Source: CAD feature listing. Evaluate the final solid. Frame: model axes, mm. Face numbers are marked on the shaded views. A direction names the side the tool comes from. Give positions to 0.01 mm unless a question says otherwise; leave off trailing zeros. Order: outer loops, then holes, each group sorted by start corner. A loop starts at its lowest first (then second) coordinate and runs counter-clockwise, first axis right, second up.
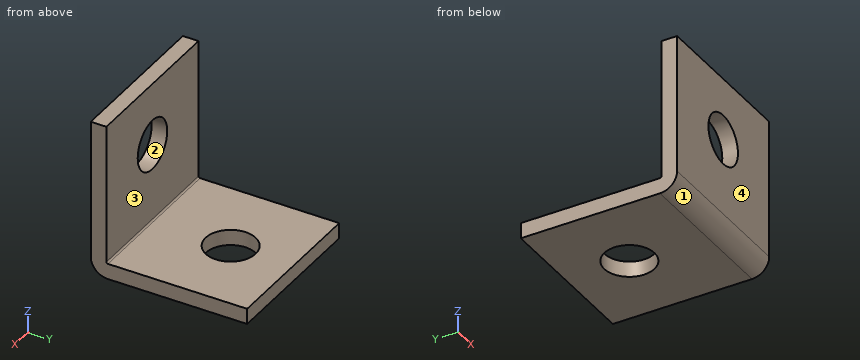
Autodesk Inventor part; units mm, degrees
ref_plane "YZ Plane" through (0, 0, 0) normal (1, 0, 0) x (0, 1, 0)
ref_plane "XZ Plane" through (0, 0, 0) normal (0, 1, 0) x (-1, 0, 0)
ref_plane "XY Plane" through (0, 0, 0) normal (0, 0, 1) x (1, 0, 0)
sketch "Sketch1" plane through (0, 0, 0) normal (0, 0, 1) x (1, 0, 0)
  line L0 (-5, 5) -> (5, 5)
  line L1 (5, 5) -> (5, -5)
  line L2 (5, -5) -> (-5, -5)
  line L3 (-5, -5) -> (-5, 5)
  line L4 (-5, 5) -> (5, -5) construction
  line L5 (5, 5) -> (-5, -5) construction
  circle A0 centre (0, 1) radius 1.6
  point P0 (0, 0)
  dimension "d0" = 10
  dimension "d1" = 10
  dimension "d3" = 3.2
  dimension "d21" = 4
extrude "Plate1" add sketch "Sketch1" along normal blind 1
sketch "Sketch2" plane through (5, -4, 0) normal (0, -1, 0) x (1, 0, 0)
  line L0 (-10, 0) -> (0, 0)
  line L1 (0, 0) -> (0, 10)
  line L2 (0, 10) -> (-10, 10)
  line L3 (-10, 10) -> (-10, 0)
edge flange "Flange1" height 10 angle 90 thickness 1 bend radius 0.1 thickness toward (0, -1, 0) relief tear relief width 1 relief depth 0.5 edges at (0, -5, 1) wall of the first edge with corners at (-5, -4, 0) (5, -4, 0) (5, -4, 10) (-5, -4, 10)
bend "Bend1"
corner "Corner1"
sketch "Sketch3" plane through (-5, -4, 10) normal (0, 1, 0) x (1, 0, 0)
  circle A0 centre (5, 4) radius 1.6
  line L0 (0, 9) -> (10, 9)
  line L1 (0, 0) -> (10, 0)
  point P0 (5, 10)
  point P1 (5, 0)
  dimension "d17" = 3.2
  dimension "d22" = 4
extrude "Cut1" cut sketch "Sketch3" against normal blind 1
equation "\"d19\" = 厚度"
equation "\"d6\" = 厚度"
equation "\"d7\" = 折彎離隙寬度"
equation "\"d8\" = 折彎離隙深度"
equation "\"d9\" = 最小剩餘"
equation "\"d10\" = 轉移半徑"
equation "\"d14\" = 轉角離隙大小"
equation "\"d15\" = 間隙大小"
equation "\"d16\" = Jacobi半徑大小"
equation "\"折彎半徑\" = 厚度"
equation "\"折彎離隙寬度\" = 厚度"
equation "\"折彎離隙深度\" = 0.5 * 厚度"
equation "\"轉角離隙大小\" = 4 * 厚度"
equation "\"最小剩餘\" = 2 * 厚度"
equation "\"轉移半徑\" = 折彎半徑"
equation "\"Jacobi半徑大小\" = 折彎半徑"
equation "\"間隙大小\" = 厚度"
properties part number "connector"
(1) Pin query (flat end, axial travel): pin 1 Ø1.5 at (x, y) = (0.5, 2) entering from +Z. Return the tip coordinate at first contact, or that it passes through.
(2) Draft query along X for the marked faces 1 and 2. Return one class per face: +X half, -X half, draft (parallel to the pull), parting line (faces both ways), or undercut.
(3) Section A-A, the plane y = 1. Return loops of the section in (x, z).
(4) Access query for the marked faces 3 and 4. Directions: +Z, -Z, +X, -X, +Y, -Y. A direction counts if a zero-diameter tool reaches every point of the face in a straight line with its end or side. Return the directions, or none.
(5) Line query: line 1 along Y through (x, z) = (1, 9.75); line 2 along Z through (x, y) = (3, -3.75); line 3 along X through (y, z) = (-4.3, 6). Output: solid intervals per line, ascending.
(6) Section C-C, the plane x = 0. Return loops of the section in (y, z).
(7) Section D-D, the plane x = 2.5. Return loops of the section in (y, z).
(8) Section B-B, the plane z = 6. Return loops of the section in (x, y).
Checks:
1. pin 1: stops at z = 1
2. face 1: draft
2. face 2: undercut
3. outline: (-5, 0) - (-1.6, 0) - (-1.6, 1) - (-5, 1) - close; (1.6, 0) - (5, 0) - (5, 1) - (1.6, 1) - close
4. face 3: +Z, +X, -X, +Y
4. face 4: +Z, -Z, +X, -X, -Y
5. line 1: y = -5 to -4
5. line 2: z = 0 to 1
5. line 3: x = -5 to -1.6, 1.6 to 5
6. outline: (-5, 1.1) arc R1.1 ccw to (-3.9, 0) - (-0.6, 0) - (-0.6, 1) - (-3.9, 1) arc R0.1 cw to (-4, 1.1) - (-4, 4.4) - (-5, 4.4) - close; (-5, 7.6) - (-4, 7.6) - (-4, 10) - (-5, 10) - close; (2.6, 0) - (5, 0) - (5, 1) - (2.6, 1) - close
7. outline: (-5, 1.1) arc R1.1 ccw to (-3.9, 0) - (5, 0) - (5, 1) - (-3.9, 1) arc R0.1 cw to (-4, 1.1) - (-4, 10) - (-5, 10) - close
8. outline: (-5, -5) - (-1.6, -5) - (-1.6, -4) - (-5, -4) - close; (1.6, -5) - (5, -5) - (5, -4) - (1.6, -4) - close
